Autodesk Inventor part; units mm, degrees
ref_plane "YZ Plane" through (0, 0, 0) normal (1, 0, 0) x (0, 1, 0)
ref_plane "XZ Plane" through (0, 0, 0) normal (0, 1, 0) x (-1, 0, 0)
ref_plane "XY Plane" through (0, 0, 0) normal (0, 0, 1) x (1, 0, 0)
sketch "Sketch2" plane through (0, 0, 0) normal (0, 1, 0) x (-1, 0, 0)
  line L0 (0, 0) -> (-15, 0)
  line L1 (-15, 0) -> (-15, 220)
  line L2 (-15, 220) -> (0, 220)
  line L3 (0, 220) -> (0, 0)
  circle A0 centre (-5, 30) radius 2.25
  circle A1 centre (-5, 190) radius 2.25
  circle A2 centre (-7.5, 50) radius 0.95
  circle A3 centre (-7.5, 90) radius 0.95
  circle A4 centre (-7.5, 130) radius 0.95
  circle A5 centre (-7.5, 170) radius 0.95
  dimension "d92" = 10
  dimension "d76" = 15
  dimension "d78" = 30
  dimension "d80" = 5
  dimension "d81" = 4.5
  dimension "d82" = 30
  dimension "d83" = 220
  dimension "d84" = 1.9
  dimension "d85" = 7.5
  dimension "d86" = 20
  dimension "d89" = 40
extrude "Extrusion2" add sketch "Sketch2" along normal blind 6
properties part number "phone_holder_botom_insert" material "Acrylic, Clear"
Model file for the job. Use its own axes, mm. Round coordinates to 2 decimals unless told otherwise and drop trailing zeros. Loops run counter-clockwise (first coordinate to the right, second up) from the corner with the lowest first, then second, coordinate; pieces in that order, holes last.
1. Wall check: probe 1 along Z at (x, y) = (7.5, 2.4); probe 2 along Z at (x, y) = (5, 3.55); probe 3 along X at (y, z) = (2.8, 130). Give the ranges that are in metal, low to high.
Check values:
probe 1: z = 0 to 49.05, 50.95 to 89.05, 90.95 to 129.05, 130.95 to 169.05, 170.95 to 220
probe 2: z = 0 to 27.75, 32.25 to 187.75, 192.25 to 220
probe 3: x = 0 to 6.55, 8.45 to 15
2. Mould opens along Z. For faces 1 (the cylindrical face through (5.488, 2.958, 192.196)), 2 (the flat face through (7, 3, 0)), 3 (the flat face through (8, 3, 220)), 4 (the flat face through (8, 0, 112)) say: +Z half, -Z half, draft (parallel to the pull), parting line (faces both ways), or undercut.
Check values:
face 1: undercut
face 2: -Z half
face 3: +Z half
face 4: draft
3. Band-saw the part on A-A, the plane z = 30. List the corners of the cut face in (x, y).
Check values:
outline: (0, 0) - (2.75, 0) - (2.75, 6) - (0, 6) - close; (7.25, 0) - (15, 0) - (15, 6) - (7.25, 6) - close
